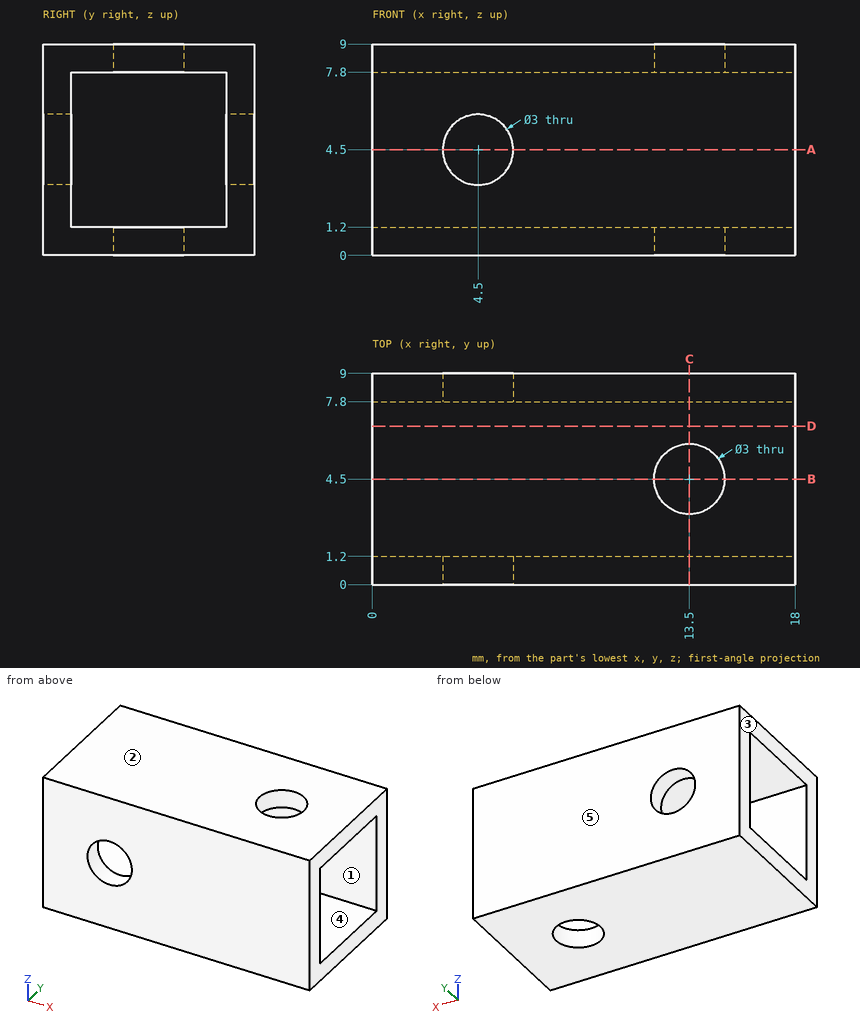
Answer from the drawing. Dimensions are ordinates in mm from the lowest x, y and z of the part. A direction names the side the tool comes from. Round coordinates to 2 decimals unless told otherwise and drop trailing zeros. Order: outer loops, then holes, each group sorted by start corner. A loop starts at its lowest first (then second) coordinate and runs counter-clockwise, first axis right, second up.
1) The part is cut by section B-B on y = 4.5. Write down the section's boundary in (x, z), plus the area to 3 significant figures.
2) The mould has two halves that part along Z. Classify the marked faces 1, 2 and 3: released by +Z, released by -Z, zero draft, split by the parting line, or undercut.
3) A flat-ended cylindrical pin translates along its axis: pin 1 (2.5 mm diameter, centred on x = 4.5, z = 4.5, fed in from +Y). Find the tip coordinate at first contact, or state that the pin passes through.
4) The part is cut by section D-D on y = 6.75. Write down the section's boundary in (x, z).
5) Straight lines are drawn through the part: L1, parallel to Z at x = 15.75, y = 4; L2, parallel to X at y = 4.5, z = 0.8. For each, find the intervals that lie inside material, in ascending order.
6) For the marked faces 4 and 5, determine the directions among +Z, -Z, +X, -X, +Y, -Y from which every point of the face is accessible in a straight line to the end or side of a thin tool.
7) The part is cut by section C-C on x = 13.5. Write down the section's boundary in (y, z), plus the area to 3 significant figures.
8) The part is cut by section A-A on z = 4.5. Write down the section's boundary in (x, y), plus the area to 3 significant figures.
Resolved:
1. outline: (0, 0) - (12, 0) - (12, 1.2) - (0, 1.2) - close; (0, 7.8) - (12, 7.8) - (12, 9) - (0, 9) - close; (15, 0) - (18, 0) - (18, 1.2) - (15, 1.2) - close; (15, 7.8) - (18, 7.8) - (18, 9) - (15, 9) - close
1. area: 36.0 mm2
2. face 1: undercut
2. face 2: released by +Z
2. face 3: zero draft
3. pin 1: passes through
4. outline: (0, 0) - (18, 0) - (18, 1.2) - (0, 1.2) - close; (0, 7.8) - (18, 7.8) - (18, 9) - (0, 9) - close
5. L1: z = 0 to 1.2, 7.8 to 9
5. L2: x = 0 to 12, 15 to 18
6. face 4: +X, -X
6. face 5: +Z, -Z, +X, -X, +Y
7. outline: (0, 0) - (3, 0) - (3, 1.2) - (1.2, 1.2) - (1.2, 7.8) - (3, 7.8) - (3, 9) - (0, 9) - close; (6, 0) - (9, 0) - (9, 9) - (6, 9) - (6, 7.8) - (7.8, 7.8) - (7.8, 1.2) - (6, 1.2) - close
7. area: 30.2 mm2
8. outline: (0, 0) - (3, 0) - (3, 1.2) - (0, 1.2) - close; (0, 7.8) - (3, 7.8) - (3, 9) - (0, 9) - close; (6, 0) - (18, 0) - (18, 1.2) - (6, 1.2) - close; (6, 7.8) - (18, 7.8) - (18, 9) - (6, 9) - close
8. area: 36.0 mm2
